```python
from build123d import *

# Parameters (mm, degrees)
SKETCH1_W           = 100
SKETCH1_H           = 100
BOSS_EXTRUDE1_DEPTH = 10
SKETCH2_R           = 4.005
CUT_EXTRUDE1_DEPTH  = 7
SKETCH3_R           = 1.65
CUT_EXTRUDE2_DEPTH  = 72.414284285
SKETCH4_OUTSIDE_W   = 130.354
SKETCH4_OUTSIDE_H   = 130.354
SKETCH4_OUTSIDE_W_2 = 69
SKETCH4_OUTSIDE_H_2 = 84.5
CUT_EXTRUDE3_DEPTH  = 72.414284285
FILLET1_R           = 20
FILLET2_SIZE        = 33
FILLET2_SIZE_2      = 60


with BuildPart() as part:
    # Sketch1 → Boss-Extrude1 (new body)
    with BuildSketch(Plane(origin=(0, 0, 0), x_dir=(1, 0, 0), z_dir=(0, 1, 0))):
        Rectangle(SKETCH1_W, SKETCH1_H)
    extrude(amount=BOSS_EXTRUDE1_DEPTH)

    # Sketch2 → Cut-Extrude1 (cut)
    with BuildSketch(Plane.XZ):
        with Locations(Location((-26.5, 28.5, 0), (0, 0, 270))):
            Circle(SKETCH2_R)
        with Locations(Location((26.5, 28.5, 0), (0, 0, 270))):
            Circle(SKETCH2_R)
        with Locations(Location((0, -26.5, 0), (0, 0, 270))):
            Circle(SKETCH2_R)
    extrude(amount=-CUT_EXTRUDE1_DEPTH, mode=Mode.SUBTRACT)

    # Sketch3 → Cut-Extrude2 (cut, through all)
    with BuildSketch(Plane(origin=(0, 10, 0), x_dir=(1, 0, 0), z_dir=(0, 1, 0))):
        with Locations(Location((-11.75, 20, 0), (0, 0, 270))):
            Circle(SKETCH3_R)
        with Locations(Location((11.75, 20, 0), (0, 0, 270))):
            Circle(SKETCH3_R)
        with Locations(Location((11.75, -13, 0), (0, 0, 270))):
            Circle(SKETCH3_R)
        with Locations(Location((18, -40, 0), (0, 0, 270))):
            Circle(SKETCH3_R)
        with Locations(Location((-18, -40, 0), (0, 0, 270))):
            Circle(SKETCH3_R)
        with Locations(Location((-11.75, -13, 0), (0, 0, 270))):
            Circle(SKETCH3_R)
    extrude(amount=-CUT_EXTRUDE2_DEPTH, mode=Mode.SUBTRACT)

    # Sketch4 outside → Cut-Extrude3 (cut, through all)
    with BuildSketch(Plane(origin=(0, 10, 0), x_dir=(1, 0, 0), z_dir=(0, 1, 0))):
        Rectangle(SKETCH4_OUTSIDE_W, SKETCH4_OUTSIDE_H)
        with Locations((0, -7.75)):
            Rectangle(SKETCH4_OUTSIDE_W_2, SKETCH4_OUTSIDE_H_2, mode=Mode.SUBTRACT)
    extrude(amount=-CUT_EXTRUDE3_DEPTH, mode=Mode.SUBTRACT)

    # Fillet1
    fillet1_edges = [part.edges().sort_by_distance(p)[0] for p in [
        (-34.5, 5, 50),
        (34.5, 5, 50),
    ]]
    fillet(fillet1_edges, radius=FILLET1_R)

    # Fillet2
    # an asymmetric fillet: 60, 33 mm, written as the material it takes off along each edge
    with BuildSketch(Plane(origin=(34.5, 160, -34.5), x_dir=(-1, 0, 0), z_dir=(0, -1, 0))) as fillet2_piece_1:
        with BuildLine():
            Bezier((FILLET2_SIZE, 0), (0, 0), (0, -FILLET2_SIZE_2), weights=[1, 0.707106781, 1])
            Line((0, -FILLET2_SIZE_2), (0, 0))
            Line((0, 0), (FILLET2_SIZE, 0))
        make_face()
    extrude(amount=310, mode=Mode.SUBTRACT)
    with BuildSketch(Plane(origin=(-34.5, 160, -34.5), x_dir=(0, 0, 1), z_dir=(0, -1, 0))) as fillet2_piece_2:
        with BuildLine():
            Bezier((FILLET2_SIZE_2, 0), (0, 0), (0, -FILLET2_SIZE), weights=[1, 0.707106781, 1])
            Line((0, -FILLET2_SIZE), (0, 0))
            Line((0, 0), (FILLET2_SIZE_2, 0))
        make_face()
    extrude(amount=310, mode=Mode.SUBTRACT)


solid = part.part
```
CAD build for the part. Positions are in the model's coordinates, mm. A direction names the side the tool comes from. Coordinates: 2 decimals unless noted, no trailing zeros. Write each loop counter-clockwise with the first axis right and the second up, starting at its lowest first coordinate (ties: lowest second). Pieces come first, ordered by that corner, then holes.
(1) Cut at B-B, the plane z = 28.5. List the corners of the cut face in (x, y) (3 decimals).
(2) Drill centre lines: probe 1 along X at (y, z) = (4.5, 28.5) (3 decimals); probe 2 along Z at (x, y) = (12, 4.25); probe 3 along X at (y, z) = (1.5, 26.5). Where is each one in solid material? Low to high.
(3) 3-axis set-ups, long thin cutter, end or side, ignore diameter. For faces 4 (the face through (-26, 7, 29)), 5 (the face through (28.486, 4.93, 44.297)): which of +Z, -Z, +X, -X, +Y, -Y reach the whole face in a straight line?
(4) Flat gauge pins, fed straight in: pin 1 (6.5 mm diameter, centred on x = -27, z = 28.5, fed in from -Y); pin 2 (2.5 mm diameter, centred on x = -11.75, z = -20, fed in from +Y); pin 3 (5 mm diameter, centred on y = 3, z = 40, fed in from +X). Where does each tip first touch, or does it go through?
(5) Two-plate mould, pull along X, no slides. Class faces 1 (the face through (0, 10, 17)), 2 (the face through (-17.93, 5.07, 38.35)), 3 (the face through (-34.5, 5, 28)): +X half, -X half, draft (parallel to the pull), parting line (faces both ways), or undercut.
(6) Cut at A-A, the plane x = 0. List the corners of the cut face in (y, z) (3 decimals).
(7) Cut at C-C, the plane y = 1.5. Count the separate pieces of the cut face and the enclosed holes in it, and give its area (3 significant figures).
Geometry says:
1. outline: (-34.5, 0) - (-30.505, 0) - (-30.505, 7) - (-22.495, 7) - (-22.495, 0) - (22.495, 0) - (22.495, 7) - (30.505, 7) - (30.505, 0) - (34.5, 0) - (34.5, 10) - (-34.5, 10) - close
2. probe 1: x = -34.5 to -30.505, -22.495 to 22.495, 30.505 to 34.5
2. probe 2: z = -31.38 to -21.63, -18.37 to 11.37, 14.63 to 50
2. probe 3: x = -34.5 to -29.97, -23.03 to 23.03, 29.97 to 34.5
3. face 4: -Y
3. face 5: +Z, +X, +Y, -Y
4. pin 1: stops at y = 7
4. pin 2: passes through
4. pin 3: stops at x = 33.04
5. face 1: draft
5. face 2: undercut
5. face 3: -X half
6. outline: (0, -34.5) - (10, -34.5) - (10, 50) - (0, 50) - (0, -22.495) - (7, -22.495) - (7, -30.505) - (0, -30.505) - close
7. separate pieces: 1
7. enclosed holes: 9
7. area: 4,610 mm2
